Verification items for this drawing (mm, ordinates from the low corner). Coordinates: 2 decimals unless noted, no trailing zeros. Loops run counter-clockwise (first coordinate to the right, second up) from the corner with the lowest first, then second, coordinate; pieces in that order, holes last. Notation, with made-up numbers: M -39,24 L 17,24 A15 cw 17,42 Z; hole C 32,0.5 d10. An arc over 180 degrees is marked long. Use CSV: the item, a comma, the result in double quotes.
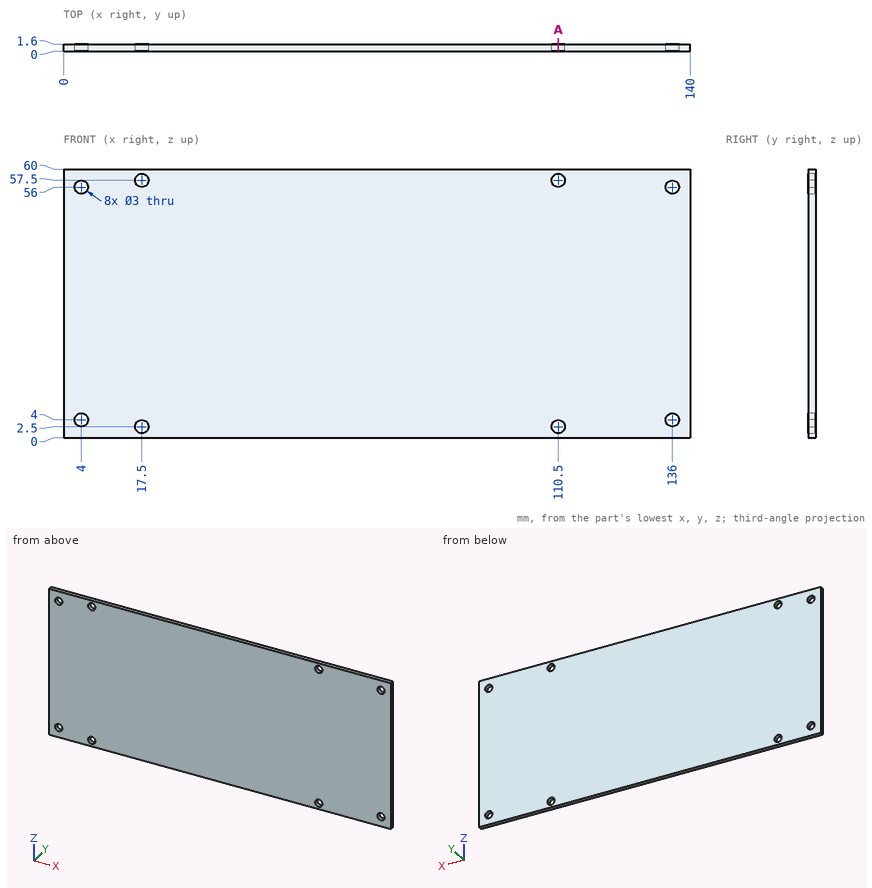
1. Thickness scan on line 1 (Z direction, x = 136, y = 1.2); line 2 (Z direction, x = 110.5, y = 0.9); line 3 (X direction, y = 1, z = 3.5). Record the ranges inside material, lowest first. Write a range as [from, to].
The answers:
line 1,"[0, 2.5], [5.5, 54.5], [57.5, 60]"
line 2,"[0, 1], [4, 56], [59, 60]"
line 3,"[0, 2.59], [5.41, 16.38], [18.62, 109.38], [111.62, 134.59], [137.41, 140]"
2. Section check A-A, the plane x = 110.5. Record the cut outline in (y, z), plus the area to 3 significant figures.
The answers:
outline,"M 0,0 L 1.6,0 L 1.6,1 L 0,1 Z; M 0,4 L 1.6,4 L 1.6,56 L 0,56 Z; M 0,59 L 1.6,59 L 1.6,60 L 0,60 Z"
area,"86.4 mm^2"
3. Gauge pin test, flat end, axial feed: P1, Ø2.5, axis at x = 110.5, z = 57.5, coming from the +Y side. Record the tip position at first contact, or that the pin passes through.
The answers:
P1,"through"
